```python
from build123d import *

# Parameters (mm, degrees)
SKETCH1_W                                        = 50
SKETCH1_H                                        = 25
BOSS_EXTRUDE1_DEPTH                              = 20
CBORE_FOR_M4_HEX_HEAD_MACHINE_SCREW1_D           = 4.5
CBORE_FOR_M4_HEX_HEAD_MACHINE_SCREW1_CBORE_D     = 8
CBORE_FOR_M4_HEX_HEAD_MACHINE_SCREW1_CBORE_DEPTH = 6
F_4_0_4_DIAMETER_HOLE1_D                         = 4
F_4_0_4_DIAMETER_HOLE1_DEPTH                     = 29.359687576
F_4_2_4_2_DIAMETER_HOLE1_D                       = 4.2
F_4_2_4_2_DIAMETER_HOLE1_DEPTH                   = 44.692225279


with BuildPart() as part:
    # Sketch1 → Boss-Extrude1 (new body)
    with BuildSketch(Plane(origin=(0, 10, 0), x_dir=(1, 0, 0), z_dir=(0, 1, 0))):
        with Locations((0, -12.5)):
            Rectangle(SKETCH1_W, SKETCH1_H)
    extrude(amount=-BOSS_EXTRUDE1_DEPTH)

    # CBORE for M4 Hex Head Machine Screw1 (through all)
    with Locations(Plane(origin=(0, 10, 0), x_dir=(1, 0, 0), z_dir=(0, 1, 0))):
        with Locations((-12.5, -4.5), (12.5, -4.5)):
            CounterBoreHole(CBORE_FOR_M4_HEX_HEAD_MACHINE_SCREW1_D / 2, CBORE_FOR_M4_HEX_HEAD_MACHINE_SCREW1_CBORE_D / 2, CBORE_FOR_M4_HEX_HEAD_MACHINE_SCREW1_CBORE_DEPTH)

    # Ø4.0 (4) Diameter Hole1
    with Locations(Plane(origin=(0, 10, 0), x_dir=(1, 0, 0), z_dir=(0, 1, 0))):
        with Locations((-12.5, -12.5), (12.5, -12.5)):
            Hole(F_4_0_4_DIAMETER_HOLE1_D / 2, depth=F_4_0_4_DIAMETER_HOLE1_DEPTH)

    # Ø4.2 (4.2) Diameter Hole1
    with Locations(Plane(origin=(0, 0, 0), x_dir=(-1, 0, 0), z_dir=(0, 0, -1))):
        with Locations((12.5, 0), (-12.5, 0)):
            Hole(F_4_2_4_2_DIAMETER_HOLE1_D / 2, depth=F_4_2_4_2_DIAMETER_HOLE1_DEPTH)


solid = part.part
```
Geometry check sheet. Reference: the model listing, model coordinates, mm. A direction names the side the tool comes from. Round coordinates to 2 decimals unless told otherwise and drop trailing zeros. Loops run counter-clockwise (first coordinate to the right, second up) from the corner with the lowest first, then second, coordinate; pieces in that order, holes last. Notation, with made-up numbers: M 59,-39.5 L 78,-39.5 A7 ccw 78,-34.5 Z; hole C 21.5,34 d9. An arc over 180 degrees is marked long. Return JSON: item names as keys, results as strings. Group by question number.
(1) Set-up check for faces 4 (the face through (-15.7, 7, 6.9)), 5 (the face through (-10.497, 0.631, 15.292)): record each of +Z, -Z, +X, -X, +Y, -Y from which the full face is reachable in a straight line by a thin tool's end or side.
(2) Scan lines: line 1 along Z through (x, y) = (-12.5, -4.5); line 2 along X through (y, z) = (3.75, 12.5); line 3 along X through (y, z) = (0, 17.5). Record each from-to range of solid material in increasing order. Write a range as [from, to].
(3) Section check C-C, the plane y = 6.75. Enter the section's corners in (x, z).
(4) Go/stop test with flat-tipped pins: pin 1 (9 mm diameter, centred on x = 10.5, z = 3.5, fed in from +Y); pin 2 (5 mm diameter, centred on x = 12.5, z = 4.5, fed in from +Y). Record where each tip stops, or that it passes through.
(5) Mould release check, pull along Y, two halves, no side actions. Record for faces 1 (the face through (0, 0, 25)), 2 (the face through (10.834, -1.278, 1.462)), 3 (the face through (-10.8, 4, 6.2)): pulls with the +Y half, pulls with the -Y half, needs draft (parallel to the pull), parting line crosses it, or undercut.
(6) Section check A-A, the plane x = -12.5. Enter the section's corners in (y, z).
(7) Section check B-B, the plane z = 12.5. Enter the section's corners in (x, y).
(8) Section check D-D, the plane z = 19.5. Enter the section's corners in (x, y), and give its area (3 significant figures).
Data:
{
 "1": {"face 4": "+Y", "face 5": "+Z, -Z"},
 "2": {"line 1": "[0, 2.25], [6.75, 10.5], [14.5, 25]", "line 2": "[-25, -14.5], [-10.5, 10.5], [14.5, 25]", "line 3": "[-25, -14.6], [-10.4, 10.4], [14.6, 25]"},
 "3": {"outline": "M -25,0 L 25,0 L 25,25 L -25,25 Z; hole C -12.5,4.5 d8; hole C -12.5,12.5 d4; hole C 12.5,4.5 d8; hole C 12.5,12.5 d4"},
 "4": {"pin 1": "y = 10", "pin 2": "y = 4"},
 "5": {"face 1": "needs draft", "face 2": "undercut", "face 3": "pulls with the +Y half"},
 "6": {"outline": "M -10,0 L -2.1,0 L -2.1,2.25 L -10,2.25 Z; M -10,6.75 L -2.1,6.75 L -2.1,10.5 L -10,10.5 Z; M -10,14.5 L -2.1,14.5 L -2.1,25 L -10,25 Z; M 2.1,0 L 10,0 L 10,0.5 L 4,0.5 L 4,2.25 L 2.1,2.25 Z; M 2.1,6.75 L 4,6.75 L 4,8.5 L 10,8.5 L 10,10.5 L 2.1,10.5 Z; M 2.1,14.5 L 10,14.5 L 10,25 L 2.1,25 Z"},
 "7": {"outline": "M -25,-10 L -14.5,-10 L -14.5,-0.64 A2.1 cw -14.5,0.64 L -14.5,10 L -25,10 Z; M -10.5,-10 L 10.5,-10 L 10.5,-0.64 A2.1 cw 10.5,0.64 L 10.5,10 L -10.5,10 L -10.5,0.64 A2.1 cw -10.5,-0.64 Z; M 14.5,-10 L 25,-10 L 25,10 L 14.5,10 L 14.5,0.64 A2.1 cw 14.5,-0.64 Z"},
 "8": {"outline": "M -25,-10 L 25,-10 L 25,10 L -25,10 Z; hole C -12.5,0 d4.2; hole C 12.5,0 d4.2", "area": "972 mm²"}
}
